Read the model definition and answer for the solid it produces. Units are mm, in the model's axes. A direction names the side the tool comes from. Give positions to 0.01 mm unless a question says otherwise; leave off trailing zeros. Write each loop counter-clockwise with the first axis right and the second up, starting at its lowest first coordinate (ties: lowest second). Pieces come first, ordered by that corner, then holes. Notation, with made-up numbers: (63.5, 35.5) -> (120.5, 35.5) arc R13 ccw to (120.5, 56.5) -> close; hole circle Ø8 at (-18, 29.25). An arc over 180 degrees is marked (long way). Write item = value, one per line.
from build123d import *

# Parameters (mm, degrees)
BOSS_EXTRU_1_DEPTH = 2
BOSS_EXTRU_2_DEPTH = 0.5
BOSS_EXTRU_2_DRAFT = 15
BOSS_EXTRU_3_DEPTH = 1


with BuildPart() as part:
    # Esquisse1 → Boss.-Extru.1 (new body)
    with BuildSketch(Plane.XY):
        with BuildLine():
            Line((-9.75, 5), (9.75, 5))
            ThreePointArc((9.75, 5), (10.810660172, 4.560660172), (11.25, 3.5))
            Line((11.25, 3.5), (11.25, -3.5))
            ThreePointArc((11.25, -3.5), (10.810660172, -4.560660172), (9.75, -5))
            Line((9.75, -5), (-9.75, -5))
            ThreePointArc((-9.75, -5), (-10.810660172, -4.560660172), (-11.25, -3.5))
            Line((-11.25, -3.5), (-11.25, 3.5))
            ThreePointArc((-11.25, 3.5), (-10.810660172, 4.560660172), (-9.75, 5))
        make_face()
        with BuildLine():
            Line((-2.5, 1), (2.5, 1))
            ThreePointArc((2.5, 1), (3.5, 0), (2.5, -1))
            Line((2.5, -1), (-2.5, -1))
            ThreePointArc((-2.5, -1), (-3.5, 0), (-2.5, 1))
        make_face(mode=Mode.SUBTRACT)
    extrude(amount=BOSS_EXTRU_1_DEPTH)


with BuildPart() as boss_extru_2_tool:
    # Esquisse2 → Boss.-Extru.2 (with draft: the straight prism first)
    with BuildSketch(Plane.XY.offset(2)):
        with BuildLine():
            Line((-9.75, -5), (9.75, -5))
            ThreePointArc((9.75, -5), (10.810660172, -4.560660172), (11.25, -3.5))
            Line((11.25, -3.5), (11.25, 3.5))
            ThreePointArc((11.25, 3.5), (10.810660172, 4.560660172), (9.75, 5))
            Line((9.75, 5), (-9.75, 5))
            ThreePointArc((-9.75, 5), (-10.810660172, 4.560660172), (-11.25, 3.5))
            Line((-11.25, 3.5), (-11.25, -3.5))
            ThreePointArc((-11.25, -3.5), (-10.810660172, -4.560660172), (-9.75, -5))
        make_face()
        with BuildLine():
            Line((2.5, 1), (-2.5, 1))
            ThreePointArc((-2.5, 1), (-3.5, 0), (-2.5, -1))
            Line((-2.5, -1), (2.5, -1))
            ThreePointArc((2.5, -1), (3.5, 0), (2.5, 1))
        make_face(mode=Mode.SUBTRACT)
    extrude(amount=BOSS_EXTRU_2_DEPTH)
    # Boss.-Extru.2: the draft: its side faces are tilted about the plane it starts from
    boss_extru_2_sides = [boss_extru_2_tool.faces().sort_by_distance(p)[0] for p in [
        (0, -5, 2.25),
        (10.810660172, -4.560660172, 2.25),
        (11.25, 0, 2.25),
        (10.810660172, 4.560660172, 2.25),
        (0, 5, 2.25),
        (-10.810660172, 4.560660172, 2.25),
        (-11.25, 0, 2.25),
        (-10.810660172, -4.560660172, 2.25),
        (-3.5, 0, 2.25),
        (0, 1, 2.25),
        (3.5, 0, 2.25),
        (0, -1, 2.25),
    ]]
    draft(boss_extru_2_sides, Plane.XY.offset(2), BOSS_EXTRU_2_DRAFT)


with BuildPart() as part_1:
    add(part.part)

    # Boss.-Extru.2: add boss_extru_2_tool
    add(boss_extru_2_tool.part)

    # Esquisse3 → Boss.-Extru.3 (add)
    with BuildSketch(Plane(origin=(0, 0, 0), x_dir=(-1, 0, 0), z_dir=(0, 0, -1))):
        with BuildLine():
            Line((12.25, -3.5), (12.25, 3.5))
            ThreePointArc((12.25, 3.5), (11.517766953, 5.267766953), (9.75, 6))
            Line((9.75, 6), (-9.75, 6))
            ThreePointArc((-9.75, 6), (-11.517766953, 5.267766953), (-12.25, 3.5))
            Line((-12.25, 3.5), (-12.25, -3.5))
            ThreePointArc((-12.25, -3.5), (-11.517766953, -5.267766953), (-9.75, -6))
            Line((-9.75, -6), (9.75, -6))
            ThreePointArc((9.75, -6), (11.517766953, -5.267766953), (12.25, -3.5))
        make_face()
        with BuildLine():
            Line((11.25, -3.5), (11.25, 3.5))
            ThreePointArc((11.25, 3.5), (10.810660172, 4.560660172), (9.75, 5))
            Line((9.75, 5), (-9.75, 5))
            ThreePointArc((-9.75, 5), (-10.810660172, 4.560660172), (-11.25, 3.5))
            Line((-11.25, 3.5), (-11.25, -3.5))
            ThreePointArc((-11.25, -3.5), (-10.810660172, -4.560660172), (-9.75, -5))
            Line((-9.75, -5), (9.75, -5))
            ThreePointArc((9.75, -5), (10.810660172, -4.560660172), (11.25, -3.5))
        make_face(mode=Mode.SUBTRACT)
    extrude(amount=-BOSS_EXTRU_3_DEPTH)


solid = part_1.part
(1) A tool of negligible diameter and unlimited length cuts with its end or side. For faces 1 (the conical face through (-3.55, 0.02, 2.19)), 2 (the flat face through (0, -1, 1)), 3 (the cylindrical face through (-10.82, 4.55, 1.49)), 4 (the flat face through (-11.25, 0, 1.5)), 5 (the cylindrical face through (10.82, -4.55, 1.49)), from which of +Z, -Z, +X, -X, +Y, -Y can it reach the whole face along a straight path? Write none if from no direction.
Checks:
face_1 = +Z
face_2 = +Z, -Z
face_3 = +Z, -X, +Y
face_4 = +Z, -X, +Y, -Y
face_5 = +Z, +X, -Y
(2) For a pull along Y with two mould halves and no side action, classify faces 6 (the flat face through (0.1, -5, 1.5)), 7 (the flat face through (0, 1, 1)), 8 (the flat face through (-12.25, 0, 0.5)) as released by +Y, released by -Y, zero draft, split by the parting line, or undercut.
Checks:
face_6 = released by -Y
face_7 = undercut
face_8 = zero draft
(3) The part is cut by section B-B on z = 1.3. Determine the outline of the cut face in (x, y), plus the area to 3 significant figures.
Checks:
outline = (-11.25, -3.5) arc R1.5 ccw to (-9.75, -5) -> (9.75, -5) arc R1.5 ccw to (11.25, -3.5) -> (11.25, 3.5) arc R1.5 ccw to (9.75, 5) -> (-9.75, 5) arc R1.5 ccw to (-11.25, 3.5) -> close; hole (-2.5, -1) -> (2.5, -1) arc R1 ccw to (2.5, 1) -> (-2.5, 1) arc R1 ccw to start
area = 210 mm²
(4) The part is cut by section C-C on x = 6.75. Determine the outline of the cut face in (y, z).
Checks:
outline = (-6, 0) -> (6, 0) -> (6, 1) -> (5, 1) -> (5, 2) -> (4.87, 2.5) -> (-4.87, 2.5) -> (-5, 2) -> (-5, 1) -> (-6, 1) -> close
(5) The part is cut by section D-D on y = 2.5. Determine the outline of the cut face in (x, z), plus the area to 3 significant figures.
Checks:
outline = (-12.25, 0) -> (12.25, 0) -> (12.25, 1) -> (11.25, 1) -> (11.25, 2) -> (11.12, 2.5) -> (-11.12, 2.5) -> (-11.25, 2) -> (-11.25, 1) -> (-12.25, 1) -> close
area = 58.2 mm²
(6) Consider L1, parallel to Y at x = -0.25, z = 1.65; L2, parallel to Y at x = 2.25, z = 0.85; L3, parallel to Z at x = -3, y = 5.5. Determine where each line is inside the solid, lowest interval first.
Checks:
L1 = -5 to -1, 1 to 5
L2 = -6 to -1, 1 to 6
L3 = 0 to 1
(7) The part is cut by section A-A on y = 0. Determine the outline of the cut face in (x, z).
Checks:
outline = (-12.25, 0) -> (-3.5, 0) -> (-3.5, 2) -> (-3.63, 2.5) -> (-11.12, 2.5) -> (-11.25, 2) -> (-11.25, 1) -> (-12.25, 1) -> close; (3.5, 0) -> (12.25, 0) -> (12.25, 1) -> (11.25, 1) -> (11.25, 2) -> (11.12, 2.5) -> (3.63, 2.5) -> (3.5, 2) -> close
(8) Given P1, Ø0.8, axis at x = -1, z = 1.5, coming from the -Y side; P2, Ø1.1, axis at y = 1, z = 1.5, coming from the +X side, each flat-ended and moving along its own axis, determine where each tip first touches the part or whether it passes through.
Checks:
P1 = -5
P2 = 12.25
